Study the drawing (mm; zero at the part's minimum x, y, z) and answer. Round coordinates to 2 decimals unless told otherwise and drop trailing zeros. Loops run counter-clockwise (first coordinate to the right, second up) from the corner with the lowest first, then second, coordinate; pieces in that order, holes last. Notation, with made-up numbers: M 49.5,46.25 L 104.5,46.25 A28 ccw 104.5,80.25 Z; hole C 4.25,78 d11. An arc over 180 degrees is marked long. Put each result on its own line as item: value. Start each with the question number.
(1) Section A-A, the plane x = 34.5 is taken. Determine the outline of the cut face in (y, z), then the cut area to 3 significant figures.
(2) Straight lines are drawn through the part: line 1 (X direction, y = 68.5, z = 2.4); line 2 (Y direction, x = 17, z = 2.4); line 3 (Y direction, x = 39, z = 2.15) (1 decimal). For each, find the intervals that lie inside material, in ascending order.
(3) Section B-B, the plane z = 2.15 is taken. Count the separate pieces of the cut face and the enclosed holes in it, then the cut area to 3 significant figures.
(4) Flat-ended cylindrical pins translate along their axes: P1, Ø1.4, axis at x = 21.53, y = 63.09, coming from the +Z side; P2, Ø0.8, axis at y = 1.5, z = 0.5, coming from the -X side; P3, Ø1.4, axis at y = 1.5, z = 2, coming from the +X side. Find the tip coordinate at first contact, or state that the pin passes through.
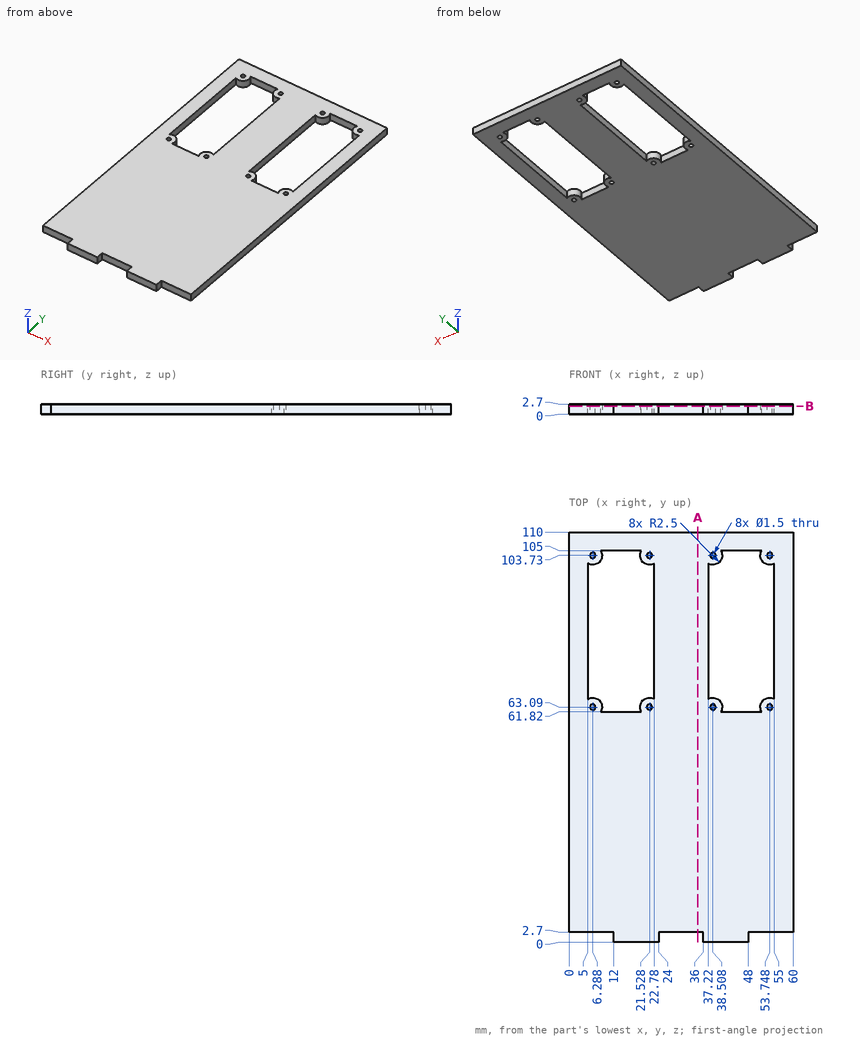
Recorded:
1. outline: M 2.7,0 L 110,0 L 110,2.7 L 2.7,2.7 Z
1. area: 290 mm²
2. line 1: x = 0 to 5, 22.78 to 37.22, 55 to 60
2. line 2: y = 0 to 61.82, 105 to 110
2. line 3: y = 0 to 62.5, 63.7 to 65.5, 101.3 to 103.2, 104.3 to 110
3. separate pieces: 1
3. enclosed holes: 10
3. area: 5,050 mm²
4. P1: passes through
4. P2: stops at x = 12
4. P3: stops at x = 48
